Read the model definition and answer for the solid it produces. Units are mm, in the model's axes. Give positions to 0.01 mm unless a question says otherwise; leave off trailing zeros. Loops run counter-clockwise (first coordinate to the right, second up) from the corner with the lowest first, then second, coordinate; pieces in that order, holes last.
(1) Determine the mould class of faces 1 (the face through (0, -5, 23)), 2 (the face through (-0.651, 0.07, 54.957)), 3 (the face through (-12.403, -0.07, 26.596)) for opening direction Z: pulls with the +Z half, pulls with the -Z half, needs draft (parallel to the pull), parting line crosses it, or undercut.
(2) Find section D-D, the plane z = 50. Write down the section's boundary in (x, y), then the cut area to 3 significant figures.
(3) Find section A-A, the plane x = 0. Write down the section's boundary in (y, z), then the cut area to 3 significant figures.
(4) Find section B-B, the plane z = 0. Write down the section's boundary in (x, y), then the cut area to 3 significant figures.
(5) Find section C-C, the plane y = -4. Write down the section's boundary in (x, z).
(6) Each of these flat-tipped pins is pushed along its axis until it touches: P1, Ø1.5, axis at x = -3, y = 2.5, coming from the +Z side; P2, Ø1.5, axis at y = -1.5, z = 28, coming from the -X side; P3, Ø1.5, axis at x = 3, y = 3.5, coming from the -Z side; P4, Ø12, axis at x = -11.5, z = 46, coming from the +Y side. Where does it stop, or does it pass through?
(7) Straight lines are drawn through the part: probe 1 along Z at (x, y) = (0, -1); probe 2 along Z at (x, y) = (1.5, -2.25); probe 3 along X at (y, z) = (4.5, 52.5). For each, find the intervals that lie inside material, in ascending order.
```python
from build123d import *

# Parameters (mm, degrees)
F0_R     = 5
F1_DEPTH = 5


with BuildPart() as f1:
    # F0 (on Front) → F1 (new body, symmetric)
    with BuildSketch(Plane.XZ):
        with BuildLine():
            ThreePointArc((10, 50), (9.9874607311, 50.5006277506), (9.9498743711, 51))
            ThreePointArc((9.9498743711, 51), (0, 60), (-9.9498743711, 51))
            ThreePointArc((-9.9498743711, 51), (-0.5006277506, 40.0125392689), (10, 50))
        make_face()
        with Locations((0, 50)):
            Circle(F0_R, mode=Mode.SUBTRACT)
        with BuildLine():
            ThreePointArc((-14.9248115566, 1.5), (0, 15), (14.9248115566, 1.5))
            Line((14.9248115566, 1.5), (9.9498743711, 51))
            ThreePointArc((9.9498743711, 51), (9.9874607311, 50.5006277506), (10, 50))
            ThreePointArc((10, 50), (-0.5006277506, 40.0125392689), (-9.9498743711, 51))
            Line((-9.9498743711, 51), (-14.9248115566, 1.5))
        make_face()
        with BuildLine():
            ThreePointArc((-14.9248115566, 1.5), (-0.7509416259, -14.9811910967), (15, 0))
            ThreePointArc((15, 0), (14.9811910967, 0.7509416259), (14.9248115566, 1.5))
            ThreePointArc((14.9248115566, 1.5), (0, 15), (-14.9248115566, 1.5))
        make_face()
        Circle(F0_R, mode=Mode.SUBTRACT)
    extrude(amount=F1_DEPTH, both=True)


solid = f1.part
```
Entries:
1. face 1: needs draft
1. face 2: undercut
1. face 3: pulls with the +Z half
2. outline: (-10.05, -5) - (-5, -5) - (-5, 5) - (-10.05, 5) - close; (5, -5) - (10.05, -5) - (10.05, 5) - (5, 5) - close
2. area: 101 mm2
3. outline: (-5, -15) - (5, -15) - (5, -5) - (-5, -5) - close; (-5, 5) - (5, 5) - (5, 45) - (-5, 45) - close; (-5, 55) - (5, 55) - (5, 60) - (-5, 60) - close
3. area: 550 mm2
4. outline: (-15, -5) - (-5, -5) - (-5, 5) - (-15, 5) - close; (5, -5) - (15, -5) - (15, 5) - (5, 5) - close
4. area: 200 mm2
5. outline: (-14.92, 1.5) arc R15 ccw (long way) to (14.92, 1.5) - (9.95, 51) arc R10 ccw to (-9.95, 51) - close; hole circle Ø10 at (0, 0); hole circle Ø10 at (0, 50)
6. P1: stops at z = 59.74
6. P2: stops at x = -12.34
6. P3: stops at z = -14.83
6. P4: stops at y = 5
7. probe 1: z = -15 to -5, 5 to 45, 55 to 60
7. probe 2: z = -14.92 to -4.77, 4.77 to 45.23, 54.77 to 59.89
7. probe 3: x = -9.68 to -4.33, 4.33 to 9.68
